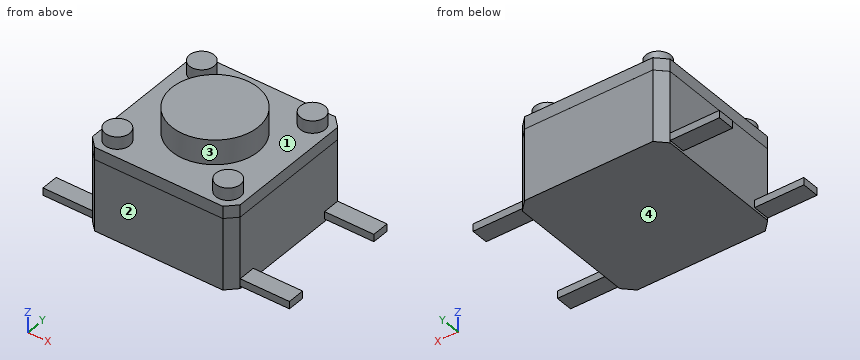
Autodesk Inventor part; units mm, degrees
ref_plane "Plano de trabajo1" through (0, 0, -3) normal (0, 0, 1) x (1, 0, 0)
ref_plane "YZ Plane" through (0, 0, 0) normal (1, 0, 0) x (0, 1, 0)
ref_plane "XZ Plane" through (0, 0, 0) normal (0, 1, 0) x (-1, 0, 0)
sketch "Boceto1" plane through (0, 0, 0) normal (0, 0, 1) x (1, 0, 0)
  line L0 (-7.8, 0) -> (4.8, 0)
  line L1 (0, -4.2) -> (0, 4.2)
  line L2 (-2.6, 3) -> (2.6, 3)
  line L3 (3, 2.6) -> (3, -2.6)
  line L4 (2.6, -3) -> (-2.6, -3)
  line L5 (-3, -2.6) -> (-3, 2.6)
  circle A0 centre (-2.25, 2.25) radius 0.5
  circle A1 centre (-2.25, -2.25) radius 0.5
  circle A2 centre (2.25, 2.25) radius 0.5
  circle A3 centre (2.25, -2.25) radius 0.5
  circle A4 centre (0, 0) radius 1.75
  line L6 (-2.6, 3) -> (-3, 2.6)
  line L7 (2.6, 3) -> (3, 2.6)
  line L8 (3, -2.6) -> (2.6, -3)
  line L9 (-3, -2.6) -> (-2.6, -3)
  point P0 (-3, 3)
  point P1 (3, -3)
  point P2 (3, 3)
  point P3 (-3, -3)
  dimension "d0" = 6
  dimension "d1" = 6
  dimension "d2" = 4.5
  dimension "d4" = 4.5
  dimension "d5" = 1
  dimension "d6" = 3.5
  dimension "d7" = 0.4
  dimension "d8" = 0.4
  dimension "d9" = 0.4
  dimension "d10" = 0.4
  dimension "d11" = 0.4
  dimension "d12" = 0.4
  dimension "d13" = 0.4
  dimension "d14" = 0.4
extrude "Extrusión1" add sketch "Boceto1" against normal blind 3.4 contours L5 L6 L2 L1 A4 L0 | L0 A4 L1 L4 L9 L5 | A4 L1 L0 | L0 L1 A4 | L1 A4 L0 | L0 A4 L1 | L1 L2 L7 L3 L0 A4 | A4 L0 L3 L8 L4 L1 | A0 | A1 | A2 | A3
extrude "Extrusión2" add sketch "Boceto1" along normal blind 0.5 contours A0 | A1 | A2 | A3
extrude "Extrusión3" add sketch "Boceto1" along normal blind 1 contours A4 L1 L0 | L0 L1 A4 | L1 A4 L0 | L0 A4 L1
ref_plane "Plano de trabajo1" through (0, 0, -3) normal (0, 0, 1) x (1, 0, 0)
sketch "Boceto2" plane through (0, 0, -3) normal (0, 0, 1) x (1, 0, 0)
  line L0 (-3, 2.6) -> (-2.6, 3)
  line L1 (-2.6, 3) -> (2.6, 3)
  line L2 (2.6, 3) -> (3, 2.6)
  line L3 (3, 2.6) -> (3, -2.6)
  line L4 (3, -2.6) -> (2.6, -3)
  line L5 (2.6, -3) -> (-2.6, -3)
  line L6 (-2.6, -3) -> (-3, -2.6)
  line L7 (-3, -2.6) -> (-3, 2.6)
  line L8 (-3, 2.6) -> (-5, 2.6)
  line L9 (-5, 2.6) -> (-5, 1.9)
  line L10 (-5, 1.9) -> (-3, 1.9)
  line L11 (-3, 1.9) -> (-3, 2.6)
  line L12 (-5, 2.25) -> (-3, 2.25)
  line L13 (-7.8, 0) -> (4.8, 0)
  line L14 (0, -4.2) -> (0, 4.2)
  line L15 (-3, -1.9) -> (-5, -1.9)
  line L16 (-5, -1.9) -> (-5, -2.6)
  line L17 (-5, -2.6) -> (-3, -2.6)
  line L18 (-3, -2.6) -> (-3, -1.9)
  line L19 (5, 2.6) -> (3, 2.6)
  line L20 (3, 2.6) -> (3, 1.9)
  line L21 (3, 1.9) -> (5, 1.9)
  line L22 (5, 1.9) -> (5, 2.6)
  line L23 (5, -1.9) -> (3, -1.9)
  line L24 (3, -1.9) -> (3, -2.6)
  line L25 (3, -2.6) -> (5, -2.6)
  line L26 (5, -2.6) -> (5, -1.9)
  point P0 (0, 0)
  point P1 (-5, -2.25)
  point P2 (-3, -2.25)
  point P3 (3, 2.25)
  point P4 (5, 2.25)
  point P5 (3, -2.25)
  point P6 (5, -2.25)
  dimension "d22" = 2
  dimension "d23" = 0.7
  dimension "d24" = 0.75
  dimension "d27" = 4.5
  dimension "d30" = 8
extrude "Extrusión4" add sketch "Boceto2" against normal blind 0.3 contours L7 L12 L9 L8 | L7 L10 L9 L12 | L19 L22 L21 L3 | L7 L17 L16 L15 | L23 L26 L25 L3
sketch "Boceto3" plane through (-2.6, 3, 0) normal (0, 1, 0) x (1, 0, 0)
  line L0 (5.2, 0) -> (0, 0)
  line L1 (5.2, 0) -> (5.2, 3.4)
  line L2 (0, 3.4) -> (5.2, 3.4)
  line L3 (0, 0) -> (0, 3.4)
  line L4 (5.2, 0.5) -> (0, 0.5)
  line L5 (0, 0) -> (0, 3.4)
  point P0 (2.6, 0)
  dimension "d35" = 0.5
extrude "Extrusión5" add sketch "Boceto3" along normal blind 0.0001 contours L0 L3 L4 L1
mirror "Simetría1" about plane through (0, 0, 0) normal (0, 1, 0) of "Extrusión5"
sketch "Boceto4" plane through (3, -2.6, 0) normal (1, 0, 0) x (0, 0, -1)
  line L0 (3.3, 5.2) -> (3.3, 4.5)
  line L1 (3.3, 4.5) -> (3, 4.5)
  line L2 (3, 4.5) -> (3, 5.2)
  line L3 (0, 5.2) -> (3, 5.2)
  line L4 (0, 0) -> (0, 5.2)
  line L5 (0, 0) -> (3, 0)
  line L6 (3, 0) -> (3, 0.7)
  line L7 (3, 0.7) -> (3.3, 0.7)
  line L8 (3.3, 0.7) -> (3.3, 0)
  line L9 (3.3, 0) -> (3.4, 0)
  line L10 (3.4, 5.2) -> (3.4, 0)
  line L11 (3.3, 5.2) -> (3.4, 5.2)
  line L12 (0.5, 0) -> (0.5, 5.2)
  point P0 (0, 2.6)
  dimension "d38" = 0.5
extrude "Extrusión6" add sketch "Boceto4" along normal blind 0.0001 contours L12 L5 L4 L3
mirror "Simetría2" about plane through (0, 0, 0) normal (1, 0, 0) of "Extrusión6"
sketch "Boceto5" plane through (3, -2.6, -3) normal (0.7071, -0.7071, 0) x (-0.7071, -0.7071, 0)
  line L0 (0.5657, -2.5) -> (0, -2.5)
  line L1 (0, -2.5) -> (0, -3)
  line L2 (0, -3) -> (0, -2.5)
  line L3 (0, -3) -> (0.5657, -3)
  line L4 (0.5657, -3) -> (0, -3)
  line L5 (0.5657, -3) -> (0.5657, -2.5)
  line L6 (0.5657, -3) -> (0.5657, -2.5)
  point P0 (0.2828, -3)
extrude "Extrusión7" add sketch "Boceto5" along normal blind 0.0001
sketch "Boceto6" plane through (3, 2.6, -3.3) normal (0.7071, 0.7071, 0) x (-0.7071, 0.7071, 0)
  line L0 (-0.0001, 3.3) -> (0.5657, 3.3)
  line L1 (0.5657, 3.3) -> (0, 3.3)
  line L2 (0.5658, 3.3) -> (0.5658, 2.8)
  line L3 (0.5657, 3.3) -> (0.5658, 2.8)
  line L4 (0.5658, 2.8) -> (0, 2.8)
  line L5 (0, 2.8) -> (-0.0001, 3.3)
  point P0 (0.2828, 3.3)
extrude "Extrusión8" add sketch "Boceto6" along normal blind 0.0001
sketch "Boceto7" plane through (-3, -2.6, -3) normal (-0.7071, -0.7071, 0) x (-0.7071, 0.7071, 0)
  line L0 (0, -2.5) -> (-0.5657, -2.5)
  line L1 (-0.5658, -2.5) -> (-0.5658, -3)
  line L2 (-0.5657, -2.5) -> (-0.5658, -3)
  line L3 (-0.5658, -3) -> (0, -3)
  line L4 (0, -3) -> (-0.5657, -3)
  line L5 (0, -3) -> (0, -2.5)
  point P0 (-0.2828, -3)
extrude "Extrusión9" add sketch "Boceto7" along normal blind 0.0001
sketch "Boceto8" plane through (-3, 2.6, -3.3) normal (-0.7071, 0.7071, 0) x (-0.7071, -0.7071, 0)
  line L0 (0, 3.3) -> (-0.5657, 3.3)
  line L1 (-0.5657, 3.3) -> (0, 3.3)
  line L2 (-0.5657, 3.3) -> (-0.5657, 2.8)
  line L3 (-0.5657, 2.8) -> (0, 2.8)
  line L4 (-0.5657, 2.8) -> (0, 2.8)
  line L5 (0, 2.8) -> (0, 3.3)
  line L6 (0, 3.3) -> (0, 2.8)
  point P0 (-0.2828, 3.3)
extrude "Extrusión10" add sketch "Boceto8" along normal blind 0.0001
properties part number "PZ_PushButton"
Input: part model. Units: mm. Frame: model coordinates. Face numbers are marked on the shaded views. A direction names the side the tool comes from. Round coordinates to 2 decimals unless told otherwise and drop trailing zeros. Loops run counter-clockwise (first coordinate to the right, second up) from the corner with the lowest first, then second, coordinate; pieces in that order, holes last. Notation, with made-up numbers: (25.25, 21.25) -> (31.25, 21.25) arc R16 ccw to (31.25, 47.25) -> close; hole circle Ø2 at (-35, -8.5). An arc over 180 degrees is marked (long way). Answer as a JSON object with one key per item and string values. Group by question number.
1) Draft query along X for the marked faces 1 and 2. Return one class per face: +X half, -X half, draft (parallel to the pull), parting line (faces both ways), or undercut.
2) Reachability of the marked faces 3 and 4 from +Z, -Z, +X, -X, +Y, -Y: full face, straight path, thin tool, end or side. Return the list, or none.
3) Section query D-D on z = -1.65. Output: boundary loops of the cut face in (x, y), plus the area to 3 significant figures.
4) Section query A-A on z = 0.2. Output: boundary loops of the cut face in (x, y).
5) Ray query, L1, parallel to Z at x = 0.25, y = 2.5; L2, parallel to Y at x = 3.75, z = -3.15; L3, parallel to X at y = 2.25, z = -1.45. Return the intervals inside material, ascending.
6) Pin query (flat end, axial travel): pin 1 (0.8 mm diameter, centred on x = 3.5, y = 2, fed in from -Z); pin 2 (0.8 mm diameter, centred on x = 3.5, y = 2.5, fed in from +Z); pin 3 (2 mm diameter, centred on y = -0.5, z = -2, fed in from -X). Return the tip coordinate at first contact, or that it passes through.
Reply:
{
 "1": {"face 1": "undercut", "face 2": "draft"},
 "2": {"face 3": "+Z", "face 4": "-Z, +X, -X, +Y, -Y"},
 "3": {"outline": "(-3, -2.6) -> (-2.6, -3) -> (2.6, -3) -> (3, -2.6) -> (3, 2.6) -> (2.6, 3) -> (-2.6, 3) -> (-3, 2.6) -> close", "area": "35.7 mm2"},
 "4": {"outline": "circle Ø1 at (-2.25, -2.25); circle Ø1 at (-2.25, 2.25); circle Ø3.5 at (0, 0); circle Ø1 at (2.25, -2.25); circle Ø1 at (2.25, 2.25)"},
 "5": {"L1": "z = -3.4 to 0", "L2": "y = -2.6 to -1.9, 1.9 to 2.6", "L3": "x = -3 to 3"},
 "6": {"pin 1": "stops at z = -3.3", "pin 2": "stops at z = -3", "pin 3": "stops at x = -3"}
}
